Read the model definition and answer for the solid it produces. Units are mm, in the model's axes. A direction names the side the tool comes from. Give positions to 0.01 mm unless a question says otherwise; leave off trailing zeros. Loops run counter-clockwise (first coordinate to the right, second up) from the corner with the lowest first, then second, coordinate; pieces in that order, holes last. Notation, with made-up numbers: (-8.5, -26) - (12.5, -26) arc R33 cw to (12.5, 7) - close; hole circle Ø5 at (51, 2). An arc over 180 degrees is marked (long way). Write item = value, one per line. Start each with the question number.
from build123d import *

# Parameters (mm, degrees)
SKETCH1_W           = 76.2
SKETCH1_H           = 190.5
SKETCH1_W_2         = 71.12
SKETCH1_H_2         = 185.42
EXTRUDE_THIN1_DEPTH = 30.48
SKETCH2_W           = 76.2
SKETCH2_H           = 190.5
BOSS_EXTRUDE1_DEPTH = 2.54
SKETCH4_W           = 71.12
SKETCH4_H           = 2.54
BOSS_EXTRUDE2_DEPTH = 30.48


with BuildPart() as part:
    # Sketch1 → Extrude-Thin1 (new body)
    with BuildSketch(Plane(origin=(0, 0, 0), x_dir=(1, 0, 0), z_dir=(0, 1, 0))):
        Rectangle(SKETCH1_W, SKETCH1_H)
        Rectangle(SKETCH1_W_2, SKETCH1_H_2, mode=Mode.SUBTRACT)
    extrude(amount=EXTRUDE_THIN1_DEPTH)

    # Sketch2 → Boss-Extrude1 (add)
    with BuildSketch(Plane.XZ):
        Rectangle(SKETCH2_W, SKETCH2_H)
    extrude(amount=BOSS_EXTRUDE1_DEPTH)

    # Sketch4 → Boss-Extrude2 (add)
    with BuildSketch(Plane(origin=(0, 0, 0), x_dir=(1, 0, 0), z_dir=(0, 1, 0))):
        with Locations((0, 63.5)):
            Rectangle(SKETCH4_W, SKETCH4_H)
    extrude(amount=BOSS_EXTRUDE2_DEPTH)


solid = part.part
1. A tool of negligible diameter and unlimited length cuts with its end or side. For faces 4 (the flat face through (-1, 14, -95.25)), 5 (the flat face through (0, 15, -64.77)), from which of +Z, -Z, +X, -X, +Y, -Y can it reach the whole face along a straight path? Write none if from no direction.
2. For a pull along Z with two mould halves and no side action, classify faces 1 (the flat face through (-38.1, 14, -1)), 2 (the flat face through (-1, 14, 95.25)), 3 (the flat face through (0, 15, -92.71)) as released by +Z, released by -Z, zero draft, split by the parting line, or undercut.
3. A cutting plane is placed at B-B on x = -6. Give the vertices of the cut face in (y, z).
4. A cutting plane is placed at C-C on z = -75.5. Give the vertices of the cut face in (x, y).
5. Consider line 1 along Z through (x, y) = (24, 5); line 2 along X through (y, z) = (28, -80); line 3 along Y through (x, z) = (-26, 28). Determine where each line is inside the solid, lowest interval first. Write a range as [from, to].
6. Given P1, Ø21.5, axis at x = 7.5, z = -14.5, coming from the +Y side, flat-ended and moving along its own axis, determine where the tip first touches the part or whether it passes through.
7. A cutting plane is placed at A-A on y = 6.5. Give the vertices of the cut face in (x, z).
Reply:
q1.face_4 = -Z, +X, -X, +Y, -Y
q1.face_5 = +Y
q2.face_1 = zero draft
q2.face_2 = released by +Z
q2.face_3 = undercut
q3.outline = (-2.54, -95.25) - (30.48, -95.25) - (30.48, -92.71) - (0, -92.71) - (0, -64.77) - (30.48, -64.77) - (30.48, -62.23) - (0, -62.23) - (0, 92.71) - (30.48, 92.71) - (30.48, 95.25) - (-2.54, 95.25) - close
q4.outline = (-38.1, -2.54) - (38.1, -2.54) - (38.1, 30.48) - (35.56, 30.48) - (35.56, 0) - (-35.56, 0) - (-35.56, 30.48) - (-38.1, 30.48) - close
q5.line_1 = [-95.25, -92.71], [-64.77, -62.23], [92.71, 95.25]
q5.line_2 = [-38.1, -35.56], [35.56, 38.1]
q5.line_3 = [-2.54, 0]
q6.P1 = 0
q7.outline = (-38.1, -95.25) - (38.1, -95.25) - (38.1, 95.25) - (-38.1, 95.25) - close; hole (-35.56, -92.71) - (35.56, -92.71) - (35.56, -64.77) - (-35.56, -64.77) - close; hole (-35.56, -62.23) - (35.56, -62.23) - (35.56, 92.71) - (-35.56, 92.71) - close
